Design review of the part shown in the three views and the two pictorial views. Dimensions are in mm from the part's minimum x, y and z. A direction names the side the tool comes from. Round coordinates to 2 decimals unless told otherwise and drop trailing zeros. Loops run counter-clockwise (first coordinate to the right, second up) from the corner with the lowest first, then second, coordinate; pieces in that order, holes last.
1. Consider section D-D on x = 7.5. State the section outline as (y, z) points.
2. To check wall thickness, follow line 1 along Y through (x, z) = (4.9, 3.75); line 2 along Y through (x, z) = (4.9, 2); line 3 along Z through (x, y) = (4.75, 0.5). State the ranges of each line that lie inside material, in increasing order.
3. Consider section C-C on z = 5. State the section outline as (x, y) points.
4. Draft analysis for pull direction Y (two halves, no side actions). For the marked faces 3, 4 and 5, state which applies: released by +Y, released by -Y, zero draft, split by the parting line, or undercut.
5. Tool access review of the marked faces 1 and 2: name each direction out of +Z, -Z, +X, -X, +Y, -Y from which nothing blocks a thin tool from reaching the whole face with its end or side.
6. Consider section A-A on x = 4.9. State the section outline as (y, z) points, then the cut area to 3 significant figures.
7. Clearance check with flat-ended pins moving along their axes: pin 1 Ø2 at (y, z) = (3, 3) entering from -X; pin 2 Ø5 at (x, z) = (1.5, 3) entering from -Y; pin 3 Ø3 at (x, z) = (2, 2.5) entering from -Y. State where each tip first meets the part, or that it passes through.
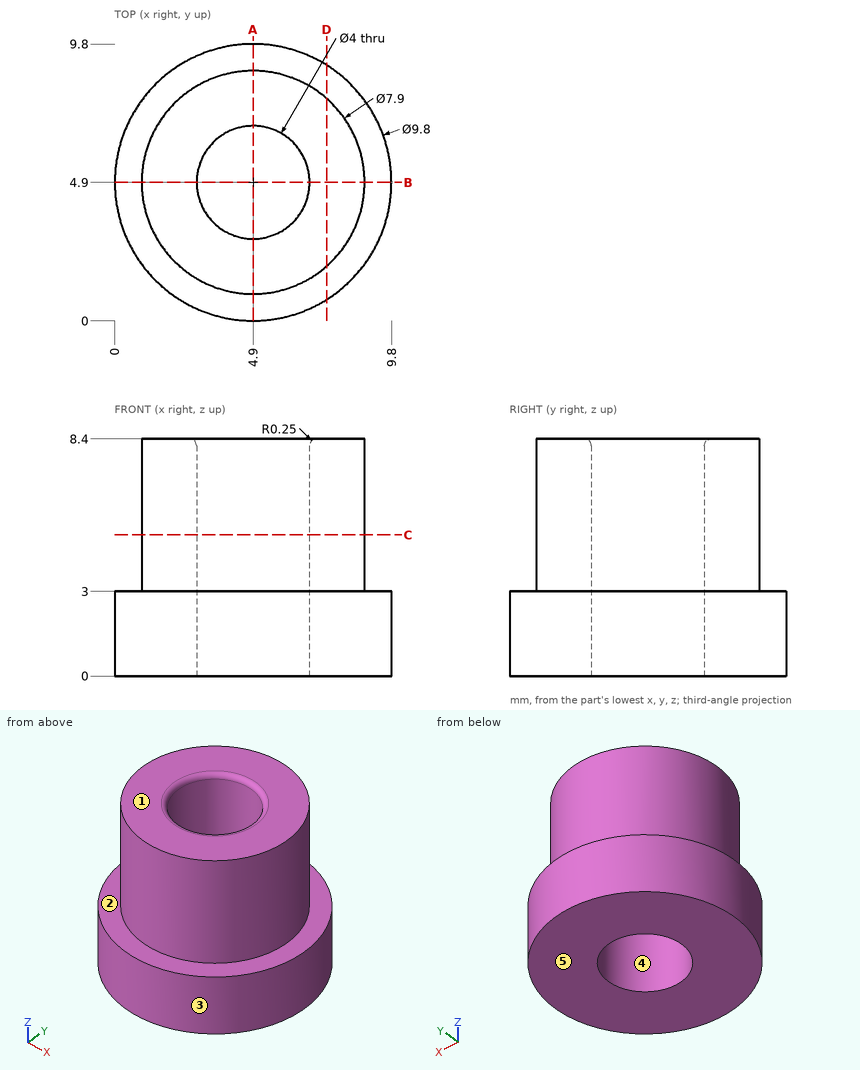
Resolved:
1. outline: (0.75, 0) - (9.05, 0) - (9.05, 3) - (7.87, 3) - (7.87, 8.4) - (1.93, 8.4) - (1.93, 3) - (0.75, 3) - close
2. line 1: y = 0.95 to 2.9, 6.9 to 8.85
2. line 2: y = 0 to 2.9, 6.9 to 9.8
2. line 3: z = 0 to 3
3. outline: circle Ø7.9 at (4.9, 4.9); hole circle Ø4 at (4.9, 4.9)
4. face 3: split by the parting line
4. face 4: undercut
4. face 5: zero draft
5. face 1: +Z, +X, -X, +Y, -Y
5. face 2: +Z
6. outline: (0, 0) - (2.9, 0) - (2.9, 8.15) arc R0.25 ccw to (2.65, 8.4) - (0.95, 8.4) - (0.95, 3) - (0, 3) - close; (6.9, 0) - (9.8, 0) - (9.8, 3) - (8.85, 3) - (8.85, 8.4) - (7.15, 8.4) arc R0.25 ccw to (6.9, 8.15) - close
6. area: 38.4 mm2
7. pin 1: stops at x = 0.08
7. pin 2: stops at y = 0.08
7. pin 3: stops at y = 0.2
